For this review, take the finished solid that the model builds, in its own axes (mm). Give positions to 0.01 mm unless a question says otherwise; leave off trailing zeros. Loops run counter-clockwise (first coordinate to the right, second up) from the corner with the lowest first, then second, coordinate; pieces in that order, holes last. Notation, with made-up numbers: M 87.5,-38 L 138.5,-38 A30 ccw 138.5,-1 Z; hole C 12.25,44.25 d2. An arc over 180 degrees is marked long. Use CSV: the item, a comma, the result in double quotes. Start each with the question number.
1. Take a section at A-A, the plane z = 12.7. Write out the cut boundary in (x, y).
2. Take a section at B-B, the plane y = 12.7. Write out the cut boundary in (x, z), and give its area (3 significant figures).
3. To check wall thickness, follow line 1 (Y direction, x = 2.65, z = 12.7); line 2 (Y direction, x = 0.7, z = 10.25); line 3 (Y direction, x = 2.5, z = 5.25). State the ranges of each line that lie inside material, in increasing order. Write a range as [from, to].
4. The part is to be moulded in two halves that separate along Z. For faces 1 (the face through (2, 39, 0)), 2 (the face through (1.972, 8.903, 5.08)), 3 (the face through (4, 39, 13)), say which applies: pulls with the +Z half, pulls with the -Z half, needs draft (parallel to the pull), parting line crosses it, or undercut.
5. Take a section at C-C, the plane x = 0.65. Write out the cut boundary in (y, z).
from build123d import *

# Parameters (mm, degrees)
SKETCH2_W                 = 4
SKETCH2_H                 = 25.4
BOSS_EXTRUDE1_DEPTH       = 80
F_4_40_TAPPED_HOLE1_D     = 2.2606
F_4_40_TAPPED_HOLE1_DEPTH = 7.6
F_4_40_TAPPED_HOLE1_TIP   = 0.679152758
SKETCH6_R                 = 3
CUT_EXTRUDE1_DEPTH        = 80


with BuildPart() as part:
    # Sketch2 → Boss-Extrude1 (new body)
    with BuildSketch(Plane(origin=(0, 0, 0), x_dir=(1, 0, 0), z_dir=(0, 1, 0))):
        with Locations((2, -12.7)):
            Rectangle(SKETCH2_W, SKETCH2_H)
    extrude(amount=BOSS_EXTRUDE1_DEPTH)

    # #4-40 Tapped Hole1
    with Locations(Plane(origin=(4, 0, 0), x_dir=(0, 0, -1), z_dir=(1, 0, 0))):
        with Locations((-12.7, 22.2), (-4.472758664, 17.45), (-4.472758664, 7.95), (-12.7, 3.2), (-20.927241336, 7.95), (-20.927241336, 17.45)):
            Hole(F_4_40_TAPPED_HOLE1_D / 2, depth=F_4_40_TAPPED_HOLE1_DEPTH)
            with Locations((0, 0, -(F_4_40_TAPPED_HOLE1_DEPTH + F_4_40_TAPPED_HOLE1_TIP / 2))):  # 118° drill point
                Cone(0, F_4_40_TAPPED_HOLE1_D / 2, F_4_40_TAPPED_HOLE1_TIP, mode=Mode.SUBTRACT)

    # Sketch6 → Cut-Extrude1 (cut)
    with BuildSketch(Plane(origin=(4, 0, 0), x_dir=(0, 0, -1), z_dir=(1, 0, 0))):
        with Locations((-12.7, 12.7)):
            Circle(SKETCH6_R)
    extrude(amount=-CUT_EXTRUDE1_DEPTH, mode=Mode.SUBTRACT)


solid = part.part
Result set:
1,outline,"M 0,0 L 4,0 L 4,2.07 L 0,2.07 Z; M 0,4.33 L 4,4.33 L 4,9.7 L 0,9.7 Z; M 0,15.7 L 4,15.7 L 4,21.07 L 0,21.07 Z; M 0,23.33 L 4,23.33 L 4,80 L 0,80 Z"
2,outline,"M 0,0 L 4,0 L 4,9.7 L 0,9.7 Z; M 0,15.7 L 4,15.7 L 4,25.4 L 0,25.4 Z"
2,area,"77.6 mm2"
3,line 1,"[0, 2.07], [4.33, 9.7], [15.7, 21.07], [23.33, 80]"
3,line 2,"[0, 10.97], [14.43, 80]"
3,line 3,"[0, 7.13], [8.77, 16.63], [18.27, 80]"
4,face 1,"pulls with the -Z half"
4,face 2,"undercut"
4,face 3,"needs draft"
5,outline,"M 0,0 L 80,0 L 80,25.4 L 0,25.4 Z; hole C 3.2,12.7 d2.26; hole C 7.95,4.47 d2.26; hole C 7.95,20.93 d2.26; hole C 12.7,12.7 d6; hole C 17.45,4.47 d2.26; hole C 17.45,20.93 d2.26; hole C 22.2,12.7 d2.26"
